CAD build for the part. Positions are in the model's coordinates, mm. Face numbers are marked on the shaded views. A direction names the side the tool comes from. Give positions to 0.01 mm unless a question says otherwise; leave off trailing zeros. Loops run counter-clockwise (first coordinate to the right, second up) from the corner with the lowest first, then second, coordinate; pieces in that order, holes last.
```python
from build123d import *

# Parameters (mm, degrees)
SKETCH1_R           = 10.125
SKETCH1_R_2         = 1.625
SKETCH1_R_3         = 2.625
BOSS_EXTRUDE1_DEPTH = 4
BOSS_EXTRUDE2_DEPTH = 10
CHAMFER1_SIZE       = 1.5


with BuildPart() as part:
    # Sketch1 → Boss-Extrude1 (new body)
    with BuildSketch(Plane(origin=(0, 0, 0), x_dir=(1, 0, 0), z_dir=(0, 1, 0))):
        with BuildLine():
            Line((-34.071067812, 11.251987552), (-39, 11.251987552))
            ThreePointArc((-39, 11.251987552), (-42.535533906, 9.787521458), (-44, 6.251987552))
            Line((-44, 6.251987552), (-44, -6.251987552))
            ThreePointArc((-44, -6.251987552), (-42.535533906, -9.787521458), (-39, -11.251987552))
            Line((-39, -11.251987552), (-34.071067812, -11.251987552))
            ThreePointArc((-34.071067812, -11.251987552), (-32.15765065, -10.871385214), (-30.535533906, -9.787521458))
            Line((-30.535533906, -9.787521458), (-28.313936139, -7.565923691))
            ThreePointArc((-28.313936139, -7.565923691), (-26.887697685, -6.508651832), (-25.159643066, -6.101457597))
            Line((-25.159643066, -6.101457597), (-24.760034307, -6.101457597))
            ThreePointArc((-24.760034307, -6.101457597), (-22.194921551, -6.923374854), (-20.585162509, -9.083010761))
            ThreePointArc((-20.585162509, -9.083010761), (-20.064123568, -10.182384075), (-19.484423936, -11.251987552))
            ThreePointArc((-19.484423936, -11.251987552), (1.21615025, -22.467108816), (20.585162509, -9.083010761))
            ThreePointArc((20.585162509, -9.083010761), (22.216290811, -6.953296816), (24.760034307, -6.101457597))
            Line((24.760034307, -6.101457597), (25.159643066, -6.101457597))
            ThreePointArc((25.159643066, -6.101457597), (26.890244586, -6.503166098), (28.313936139, -7.565923691))
            Line((28.313936139, -7.565923691), (30.535533906, -9.787521458))
            ThreePointArc((30.535533906, -9.787521458), (32.15765065, -10.871385214), (34.071067812, -11.251987552))
            Line((34.071067812, -11.251987552), (39, -11.251987552))
            ThreePointArc((39, -11.251987552), (42.535533906, -9.787521458), (44, -6.251987552))
            Line((44, -6.251987552), (44, 6.251987552))
            ThreePointArc((44, 6.251987552), (42.535533906, 9.787521458), (39, 11.251987552))
            Line((39, 11.251987552), (34.071067812, 11.251987552))
            ThreePointArc((34.071067812, 11.251987552), (32.15765065, 10.871385214), (30.535533906, 9.787521458))
            Line((30.535533906, 9.787521458), (29.212478542, 8.464466094))
            ThreePointArc((29.212478542, 8.464466094), (27.590361798, 7.380602337), (25.676944636, 7))
            Line((25.676944636, 7), (24.743686063, 7))
            ThreePointArc((24.743686063, 7), (22.08935855, 7.762719569), (20.244834052, 9.818181818))
            ThreePointArc((20.244834052, 9.818181818), (0.811483584, 22.48536178), (-19.484423936, 11.251987552))
            ThreePointArc((-19.484423936, 11.251987552), (-19.877561088, 10.541943142), (-20.244834052, 9.818181818))
            ThreePointArc((-20.244834052, 9.818181818), (-22.08935855, 7.762719569), (-24.743686063, 7))
            Line((-24.743686063, 7), (-25.676944636, 7))
            ThreePointArc((-25.676944636, 7), (-27.590361798, 7.380602337), (-29.212478542, 8.464466094))
            Line((-29.212478542, 8.464466094), (-30.535533906, 9.787521458))
            ThreePointArc((-30.535533906, 9.787521458), (-32.15765065, 10.871385214), (-34.071067812, 11.251987552))
        make_face()
        with Locations(Location((0, 0, 0), (0, 0, 270))):
            Circle(SKETCH1_R, mode=Mode.SUBTRACT)
        with Locations(Location((-12.124355653, 7, 0), (0, 0, 270))):
            Circle(SKETCH1_R_2, mode=Mode.SUBTRACT)
        with Locations(Location((12.124355653, 7, 0), (0, 0, 270))):
            Circle(SKETCH1_R_2, mode=Mode.SUBTRACT)
        with Locations(Location((0, -14, 0), (0, 0, 270))):
            Circle(SKETCH1_R_2, mode=Mode.SUBTRACT)
        with Locations(Location((-39, 7, 0), (0, 0, 270))):
            Circle(SKETCH1_R_3, mode=Mode.SUBTRACT)
        with Locations(Location((-39, -7, 0), (0, 0, 270))):
            Circle(SKETCH1_R_3, mode=Mode.SUBTRACT)
        with Locations(Location((39, -7, 0), (0, 0, 90))):
            Circle(SKETCH1_R_3, mode=Mode.SUBTRACT)
        with Locations(Location((39, 7, 0), (0, 0, 90))):
            Circle(SKETCH1_R_3, mode=Mode.SUBTRACT)
        with BuildLine():
            Line((-5.27521723, -14.493540222), (-5.923962655, -16.275953627))
            ThreePointArc((-5.923962655, -16.275953627), (-7.381618464, -17.756517255), (-9.455079093, -17.62388945))
            ThreePointArc((-9.455079093, -17.62388945), (-17.320508076, -10), (-19.990275524, 0.623606036))
            ThreePointArc((-19.990275524, 0.623606036), (-19.068404258, 2.485589517), (-17.057370639, 3.007674664))
            Line((-17.057370639, 3.007674664), (-15.189382638, 2.678297979))
            ThreePointArc((-15.189382638, 2.678297979), (-13.697315881, 1.809954494), (-13.123742589, 0.181674021))
            ThreePointArc((-13.123742589, 0.181674021), (-11.366583425, -6.5625), (-6.404536977, -11.456331486))
            ThreePointArc((-6.404536977, -11.456331486), (-5.281191369, -12.767200763), (-5.27521723, -14.493540222))
        make_face(mode=Mode.SUBTRACT)
        with BuildLine():
            Line((-9.914165408, 11.815242243), (-11.133407985, 13.268278963))
            ThreePointArc((-11.133407985, 13.268278963), (-11.686785794, 15.270927738), (-10.535196431, 17.000283414))
            ThreePointArc((-10.535196431, 17.000283414), (0, 20), (10.535196431, 17.000283414))
            ThreePointArc((10.535196431, 17.000283414), (11.686785794, 15.270927738), (11.133407985, 13.268278963))
            Line((11.133407985, 13.268278963), (9.914165408, 11.815242243))
            ThreePointArc((9.914165408, 11.815242243), (8.416124512, 10.95724627), (6.719205612, 11.274657464))
            ThreePointArc((6.719205612, 11.274657464), (0, 13.125), (-6.719205612, 11.274657464))
            ThreePointArc((-6.719205612, 11.274657464), (-8.416124512, 10.95724627), (-9.914165408, 11.815242243))
        make_face(mode=Mode.SUBTRACT)
        with BuildLine():
            Line((15.189382638, 2.678297979), (17.057370639, 3.007674664))
            ThreePointArc((17.057370639, 3.007674664), (19.068404258, 2.485589517), (19.990275524, 0.623606036))
            ThreePointArc((19.990275524, 0.623606036), (17.320508076, -10), (9.455079093, -17.62388945))
            ThreePointArc((9.455079093, -17.62388945), (7.381618464, -17.756517255), (5.923962655, -16.275953627))
            Line((5.923962655, -16.275953627), (5.27521723, -14.493540222))
            ThreePointArc((5.27521723, -14.493540222), (5.281191369, -12.767200763), (6.404536977, -11.456331486))
            ThreePointArc((6.404536977, -11.456331486), (11.366583425, -6.5625), (13.123742589, 0.181674021))
            ThreePointArc((13.123742589, 0.181674021), (13.697315881, 1.809954494), (15.189382638, 2.678297979))
        make_face(mode=Mode.SUBTRACT)
    extrude(amount=BOSS_EXTRUDE1_DEPTH)

    # Sketch2 → Boss-Extrude2 (add)
    with BuildSketch(Plane(origin=(0, 4, 0), x_dir=(1, 0, 0), z_dir=(0, 1, 0))):
        with BuildLine():
            Line((-32.6, 1.5), (-30, 1.5))
            Line((-30, 1.5), (-30, -1.5))
            Line((-30, -1.5), (-32.6, -1.5))
            ThreePointArc((-32.6, -1.5), (-33.589949494, -1.089949494), (-34, -0.1))
            Line((-34, -0.1), (-34, 0.1))
            ThreePointArc((-34, 0.1), (-33.589949494, 1.089949494), (-32.6, 1.5))
        make_face()
        with BuildLine():
            Line((-28, 1.5), (-25.4, 1.5))
            ThreePointArc((-25.4, 1.5), (-24.410050506, 1.089949494), (-24, 0.1))
            Line((-24, 0.1), (-24, -0.1))
            ThreePointArc((-24, -0.1), (-24.410050506, -1.089949494), (-25.4, -1.5))
            Line((-25.4, -1.5), (-28, -1.5))
            Line((-28, -1.5), (-28, 1.5))
        make_face()
    boss_extrude2 = extrude(amount=BOSS_EXTRUDE2_DEPTH)

    # Mirror1: Boss-Extrude2 across plane
    add(boss_extrude2.mirror(Plane(origin=(0, 0, 0), x_dir=(0, 0, 1), z_dir=(1, 0, 0))))

    # Chamfer1
    chamfer1_edges = [part.edges().sort_by_distance(p)[0] for p in [
        (-12.124355653, 4, -8.625),
        (12.124355653, 4, -8.625),
        (0, 4, 12.375),
    ]]
    chamfer(chamfer1_edges, length=CHAMFER1_SIZE)


solid = part.part
```
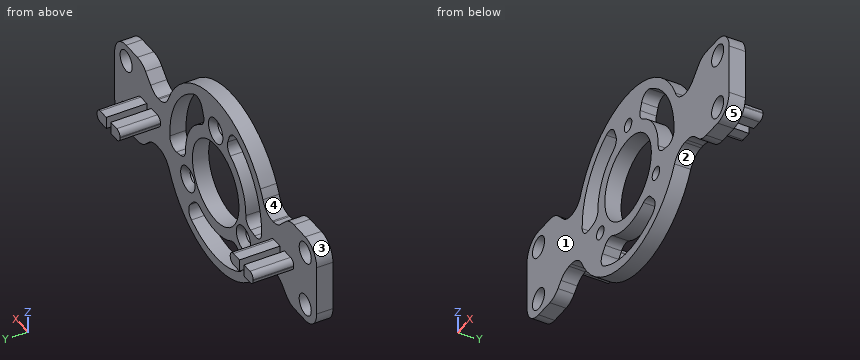
1. Tool access for the marked faces 4 and 5: list every direction of +Z, -Z, +X, -X, +Y, -Y with a clear straight run to the whole face (end or side of a thin tool).
Responses:
face 4: +Z, +Y, -Y
face 5: -Z, +X, +Y, -Y
2. Drop flat-ended pins along their axis: pin 1 (0.8 mm diameter, centred on x = -26.5, y = 11, fed in from -Z); pin 2 (3 mm diameter, centred on x = -39, z = 7, fed in from +Y); pin 3 (1.3 mm diameter, centred on x = 27, y = 6.5, fed in from +Z); pin 4 (0.9 mm diameter, centred on y = 9, z = -0.5, fed in from -X). Give the stop position or say it passes through.
Responses:
pin 1: stops at z = -1.5
pin 2: passes through
pin 3: stops at z = 1.5
pin 4: stops at x = -34
3. Saw through at B-B, the plane x = 0. List the corners of the cut face in (y, z) (3 decimals).
Responses:
outline: (0, -22.5) - (4, -22.5) - (4, -20) - (0, -20) - close; (0, -13.125) - (4, -13.125) - (4, -10.125) - (0, -10.125) - close; (0, 10.125) - (4, 10.125) - (4, 10.875) - (2.5, 12.375) - (0, 12.375) - close; (0, 15.625) - (2.5, 15.625) - (4, 17.125) - (4, 22.5) - (0, 22.5) - close
4. Saw through at D-D, the plane z = 19.5. List the corners of the cut face in (x, y).
Responses:
outline: (-11.22, 0) - (11.22, 0) - (11.22, 4) - (-11.22, 4) - close
5. Probe line 1 along Z through (x, y) = (39, 2.3) (3 decimals); line 2 along X through (y, z) = (2.1, 0) (3 decimals); line 3 along Z through (x, y) = (8, 3.25). List the from-to ranges inside material, lowest first.
Responses:
line 1: z = -11.252 to -9.625, -4.375 to 4.375, 9.625 to 11.252
line 2: x = -44 to -20, -13.125 to -10.125, 10.125 to 13.125, 20 to 44
line 3: z = -21.03 to -18.33, -10.92 to -6.21, 6.21 to 10.41, 17.91 to 21.03
6. Saw through at C-C, the plane z = 2.5. List the corners of the cut face in (x, y), and give its area (3 significant figures).
Responses:
outline: (-44, 0) - (-19.84, 0) - (-19.84, 4) - (-44, 4) - close; (-12.88, 0) - (-9.81, 0) - (-9.81, 4) - (-12.88, 4) - close; (9.81, 0) - (12.88, 0) - (12.88, 4) - (9.81, 4) - close; (19.84, 0) - (44, 0) - (44, 4) - (19.84, 4) - close
area: 218 mm2
7. Saw through at A-A, the plane y = 6. List the corners of the cut face in (x, z), and give its area (3 significant figures).
Responses:
outline: (-34, -0.1) arc R1.4 ccw to (-32.6, -1.5) - (-30, -1.5) - (-30, 1.5) - (-32.6, 1.5) arc R1.4 ccw to (-34, 0.1) - close; (-28, -1.5) - (-25.4, -1.5) arc R1.4 ccw to (-24, -0.1) - (-24, 0.1) arc R1.4 ccw to (-25.4, 1.5) - (-28, 1.5) - close; (24, -0.1) arc R1.4 ccw to (25.4, -1.5) - (28, -1.5) - (28, 1.5) - (25.4, 1.5) arc R1.4 ccw to (24, 0.1) - close; (30, -1.5) - (32.6, -1.5) arc R1.4 ccw to (34, -0.1) - (34, 0.1) arc R1.4 ccw to (32.6, 1.5) - (30, 1.5) - close
area: 44.6 mm2
8. Pull direction X, two halves, no side cores. Call the marked faces 1, 2 and 3: released by +X, released by -X, zero draft, split by the parting line, or undercut.
Responses:
face 1: zero draft
face 2: undercut
face 3: released by -X
